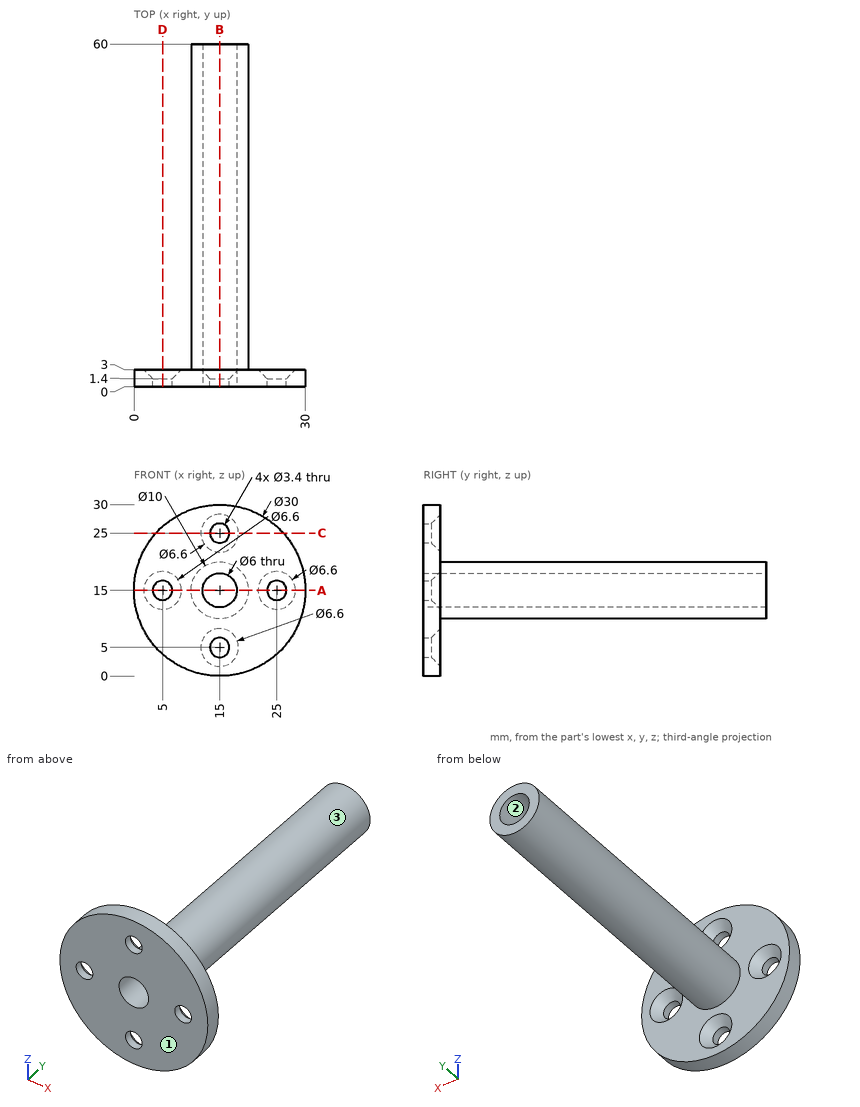
The drawing under review shows one solid part. Ordinate dimensions are in mm from its lowest x, y, z. Round coordinates to 2 decimals unless told otherwise and drop trailing zeros. Write each loop counter-clockwise with the first axis right and the second up, starting at its lowest first coordinate (ties: lowest second). Pieces come first, ordered by that corner, then holes. Notation, with made-up numbers: (77, 12) -> (132, 12) arc R33 cw to (132, 51) -> close; hole circle Ø5 at (46, 32.25). An arc over 180 degrees is marked (long way). One line per question, with ' | ' between items. Start each with the question number.
(1) Add section C-C, the plane z = 25. Write out the cut boundary in (x, y).
(2) Insertion check: P1, Ø6, axis at x = 11, y = 43, coming from the +Z side; P2, Ø4, axis at x = 15, z = 25, coming from the +Y side; P3, Ø1.5, axis at x = 19.5, y = 10, coming from the +Z side. Each pin has a flat end and moves straight along its axis. Give the tip position at first contact, or say it passes through.
(3) Add section B-B, the plane x = 15. Write out the cut boundary in (y, z).
(4) Mouldability with a two-part tool opening along Z and no side actions: class the marked faces 1, 2 and 3 as released by +Z, released by -Z, zero draft, split by the parting line, or undercut.
(5) For line 1 along X through (y, z) = (0.5, 15); line 2 along Y through (x, z) = (18, 1); line 3 along X through (y, z) = (0.45, 5), list the stretches that pass through material, from the lowest coordinate up. Write a range as from..to.
(6) Add section A-A, the plane z = 15. Write out the cut boundary in (x, y).
(7) Add section D-D, the plane x = 5. Write out the cut boundary in (y, z), plus the area to 3 significant figures.
Answer list:
1) outline: (3.82, 0) -> (13.3, 0) -> (13.3, 1.4) -> (11.7, 3) -> (3.82, 3) -> close; (16.7, 0) -> (26.18, 0) -> (26.18, 3) -> (18.3, 3) -> (16.7, 1.4) -> close
2) P1: z = 19.9 | P2: y = 1.7 | P3: z = 18.31
3) outline: (0, 0) -> (3, 0) -> (3, 1.7) -> (1.4, 3.3) -> (0, 3.3) -> close; (0, 6.7) -> (1.4, 6.7) -> (3, 8.3) -> (3, 10) -> (60, 10) -> (60, 12) -> (0, 12) -> close; (0, 18) -> (60, 18) -> (60, 20) -> (3, 20) -> (3, 21.7) -> (1.4, 23.3) -> (0, 23.3) -> close; (0, 26.7) -> (1.4, 26.7) -> (3, 28.3) -> (3, 30) -> (0, 30) -> close
4) face 1: zero draft | face 2: undercut | face 3: split by the parting line
5) line 1: 0..3.3, 6.7..12, 18..23.3, 26.7..30 | line 2: 0..3 | line 3: 3.82..13.3, 16.7..26.18
6) outline: (0, 0) -> (3.3, 0) -> (3.3, 1.4) -> (1.7, 3) -> (0, 3) -> close; (6.7, 0) -> (12, 0) -> (12, 60) -> (10, 60) -> (10, 3) -> (8.3, 3) -> (6.7, 1.4) -> close; (18, 0) -> (23.3, 0) -> (23.3, 1.4) -> (21.7, 3) -> (20, 3) -> (20, 60) -> (18, 60) -> close; (26.7, 0) -> (30, 0) -> (30, 3) -> (28.3, 3) -> (26.7, 1.4) -> close
7) outline: (0, 3.82) -> (3, 3.82) -> (3, 11.7) -> (1.4, 13.3) -> (0, 13.3) -> close; (0, 16.7) -> (1.4, 16.7) -> (3, 18.3) -> (3, 26.18) -> (0, 26.18) -> close | area: 54.3 mm²
